Input: part model. Units: mm. Frame: model coordinates. Coordinates: 2 decimals unless noted, no trailing zeros. Write each loop counter-clockwise with the first axis right and the second up, starting at its lowest first coordinate (ties: lowest second). Pieces come first, ordered by that corner, then holes.
1) Section query B-B (y = -39.5). Output: boundary loops of the cut face in (x, z).
2) Pin query (flat end, axial travel): pin 1 Ø1.6 at (y, z) = (42, 2) entering from -X; pin 2 Ø3 at (x, z) = (16.5, 2.5) entering from +Y; pin 3 Ø3 at (x, y) = (-21.5, -19) entering from -Z; pin 4 Ø1.6 at (x, z) = (26, 1.5) entering from -Y. Return the tip coordinate at first contact, or that it passes through.
3) Section query A-A (x = -23). Output: boundary loops of the cut face in (y, z), then the cut area to 3 significant figures.
4) Line query: L1, parallel to X at y = 15, z = 1.15; L2, parallel to Y at x = -18, z = 4.05; L3, parallel to X at y = -38.5, z = 4.85. Output: solid intervals per line, ascending.
from build123d import *

# Parameters (mm, degrees)
SALIENTE_EXTRUIR1_DEPTH = 5.5
CROQUIS2_W              = 26.5
CROQUIS2_H              = 5.5
CROQUIS2_W_2            = 21
SALIENTE_EXTRUIR2_DEPTH = 2.5
CROQUIS3_W              = 5.5
CROQUIS3_H              = 18.5
CROQUIS3_H_2            = 21
SALIENTE_EXTRUIR3_DEPTH = 2.5
CROQUIS4_W              = 21
CROQUIS4_H              = 5.5
CROQUIS4_W_2            = 29
SALIENTE_EXTRUIR4_DEPTH = 2.5
CROQUIS5_W              = 5.5
CROQUIS5_H              = 21
SALIENTE_EXTRUIR5_DEPTH = 2.5


with BuildPart() as part:
    # Croquis1 → Saliente-Extruir1 (new body)
    with BuildSketch(Plane.XY):
        Polygon((-57, -53.354967587), (-52.5, -53.354967587), (-52.5, -56.354967587), (-31.5, -56.354967587), (-31.5, -53.354967587), (-10.5, -53.354967587), (-10.5, -56.354967587), (10.5, -56.354967587), (10.5, -53.354967587), (31.5, -53.354967587), (31.5, -56.354967587), (52.5, -56.354967587), (52.5, -53.354967587), (73.5, -53.354967587), (73.5, -56.354967587), (94.5, -56.354967587), (100, -56.354967587), (100, -37.854967587), (97, -37.854967587), (97, -16.854967587), (100, -16.854967587), (100, 4.145032413), (97, 4.145032413), (97, 25.145032413), (100, 25.145032413), (100, 43.645032413), (73.5, 43.645032413), (73.5, 40.645032413), (52.5, 40.645032413), (52.5, 43.645032413), (31.5, 43.645032413), (31.5, 40.645032413), (10.5, 40.645032413), (10.5, 43.645032413), (-10.5, 43.645032413), (-10.5, 40.645032413), (-31.5, 40.645032413), (-31.5, 43.645032413), (-52.5, 43.645032413), (-52.5, 40.645032413), (-57, 40.645032413), (-57, 25.145032413), (-60, 25.145032413), (-60, 4.145032413), (-57, 4.145032413), (-57, -16.854967587), (-60, -16.854967587), (-60, -37.854967587), (-57, -37.854967587), align=None)
    extrude(amount=SALIENTE_EXTRUIR1_DEPTH)

    # Croquis2 → Saliente-Extruir2 (add)
    with BuildSketch(Plane(origin=(0, 43.645032413, 0), x_dir=(1, 0, 0), z_dir=(0, 1, 0))):
        with Locations((86.75, -2.75)):
            Rectangle(CROQUIS2_W, CROQUIS2_H)
        with Locations((42, -2.75)):
            Rectangle(CROQUIS2_W_2, CROQUIS2_H)
        with Locations((0, -2.75)):
            Rectangle(CROQUIS2_W_2, CROQUIS2_H)
        with Locations((-42, -2.75)):
            Rectangle(CROQUIS2_W_2, CROQUIS2_H)
    extrude(amount=SALIENTE_EXTRUIR2_DEPTH)

    # Croquis3 → Saliente-Extruir3 (add)
    with BuildSketch(Plane(origin=(100, 0, 0), x_dir=(0, 0, -1), z_dir=(1, 0, 0))):
        with Locations((-2.75, -47.104967587)):
            Rectangle(CROQUIS3_W, CROQUIS3_H)
        with Locations((-2.75, -6.354967587)):
            Rectangle(CROQUIS3_W, CROQUIS3_H_2)
        with Locations((-2.75, 35.645032413)):
            Rectangle(CROQUIS3_W, CROQUIS3_H_2)
    extrude(amount=SALIENTE_EXTRUIR3_DEPTH)

    # Croquis4 → Saliente-Extruir4 (add)
    with BuildSketch(Plane.XZ.offset(56.354967587)):
        with Locations((-42, 2.75)):
            Rectangle(CROQUIS4_W, CROQUIS4_H)
        with Locations((0, 2.75)):
            Rectangle(CROQUIS4_W, CROQUIS4_H)
        with Locations((42, 2.75)):
            Rectangle(CROQUIS4_W, CROQUIS4_H)
        with Locations((88, 2.75)):
            Rectangle(CROQUIS4_W_2, CROQUIS4_H)
    extrude(amount=SALIENTE_EXTRUIR4_DEPTH)

    # Croquis5 → Saliente-Extruir5 (add)
    with BuildSketch(Plane.ZY.offset(60)):
        with Locations((2.75, -27.354967587)):
            Rectangle(CROQUIS5_W, CROQUIS5_H)
        with Locations((2.75, 14.645032413)):
            Rectangle(CROQUIS5_W, CROQUIS5_H)
    extrude(amount=SALIENTE_EXTRUIR5_DEPTH)


solid = part.part
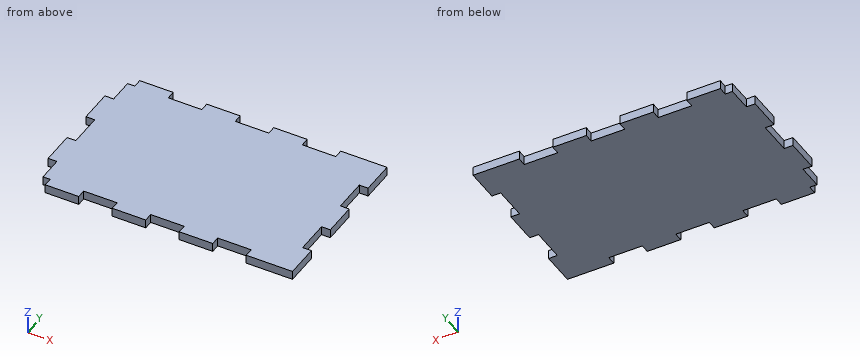
Answer:
1. outline: (-57, 0) - (102.5, 0) - (102.5, 5.5) - (-57, 5.5) - close
2. pin 1: stops at x = -52.5
2. pin 2: stops at y = 40.65
2. pin 3: stops at z = 0
2. pin 4: stops at y = -53.35
3. outline: (-53.35, 0) - (40.65, 0) - (40.65, 5.5) - (-53.35, 5.5) - close
3. area: 517 mm2
4. L1: x = -62.5 to 97
4. L2: y = -53.35 to 40.65
4. L3: x = -57 to 102.5
